from build123d import *

# Parameters (mm, degrees)
SKETCH1_R           = 12.7
BOSS_EXTRUDE1_DEPTH = 12.7
SKETCH1_3_R         = 3.175
BOSS_EXTRUDE2_DEPTH = 6.35
SKETCH1_4_R         = 3.175
BOSS_EXTRUDE3_DEPTH = 99.06


with BuildPart() as part:
    # Sketch1 → Boss-Extrude1 (new body)
    with BuildSketch(Plane.XY):
        Circle(SKETCH1_R)
    extrude(amount=-BOSS_EXTRUDE1_DEPTH)

    # Sketch1<3> → Boss-Extrude2 (add)
    with BuildSketch(Plane.XY):
        with BuildLine():
            Line((9.391776656, -58.7375), (18.783553311, -3.175))
            ThreePointArc((18.783553311, -3.175), (0, 19.05), (-18.783553311, -3.175))
            Line((-18.783553311, -3.175), (-9.391776656, -58.7375))
            ThreePointArc((-9.391776656, -58.7375), (0, -66.675), (9.391776656, -58.7375))
        make_face()
        with Locations((0, -57.15)):
            Circle(SKETCH1_3_R, mode=Mode.SUBTRACT)
    extrude(amount=BOSS_EXTRUDE2_DEPTH)

    # Sketch1<4> → Boss-Extrude3 (add)
    with BuildSketch(Plane.XY):
        with Locations((0, -57.15)):
            Circle(SKETCH1_4_R)
    extrude(amount=BOSS_EXTRUDE3_DEPTH)


solid = part.part
Design review of the part built by this model. Coordinates are the model's own, in mm. A direction names the side the tool comes from. Give positions to 0.01 mm unless a question says otherwise; leave off trailing zeros. Order: outer loops, then holes, each group sorted by start corner. A loop starts at its lowest first (then second) coordinate and runs counter-clockwise, first axis right, second up.
1. Add section A-A, the plane x = 0. State the section outline as (y, z) points (3 decimals), then the cut area to 3 significant figures.
Solution:
outline: (-66.675, 0) - (-12.7, 0) - (-12.7, -12.7) - (12.7, -12.7) - (12.7, 0) - (19.05, 0) - (19.05, 6.35) - (-53.975, 6.35) - (-53.975, 99.06) - (-60.325, 99.06) - (-60.325, 6.35) - (-66.675, 6.35) - close
area: 1,460 mm2
2. Add section B-B, the plane y = 0. State the section outline as (x, z) points, then the cut area to 3 significant figures.
Solution:
outline: (-19.05, 0) - (-12.7, 0) - (-12.7, -12.7) - (12.7, -12.7) - (12.7, 0) - (19.05, 0) - (19.05, 6.35) - (-19.05, 6.35) - close
area: 565 mm2
3. Add section C-C, the plane z = 77. State the section outline as (x, y) points (3 decimals), then the cut area to 3 significant figures.
Solution:
outline: circle Ø6.35 at (0, -57.15)
area: 31.7 mm2
4. To check wall thickness, follow L1, parallel to Z at x = 6.5, y = -62.5; L2, parallel to X at y = 1, z = 4; L3, parallel to Y at x = 4.5, z = 2. State the ranges of each line that lie inside material, in increasing order.
Solution:
L1: z = 0 to 6.35
L2: x = -19.02 to 19.02
L3: y = -65.54 to 18.51
5. Tool access review of faces 1 (the flat face through (-14.153, -30.567, 3.131)), 2 (the cylindrical face through (1.707, -54.473, 52.056)), 3 (the cylindrical face through (-2.75, -12.4, -6.26)): name each direction out of +Z, -Z, +X, -X, +Y, -Y from which nothing blocks a thin tool from reaching the whole face with its end or side.
Solution:
face 1: +Z, -Z, -X, -Y
face 2: +Z
face 3: -Z
6. Add section D-D, the plane x = 11.5. State the section outline as (y, z) points, then the cut area to 3 significant figures.
Solution:
outline: (-46.27, 0) - (-5.39, 0) - (-5.39, -12.7) - (5.39, -12.7) - (5.39, 0) - (15.19, 0) - (15.19, 6.35) - (-46.27, 6.35) - close
area: 527 mm2
7. For pin 1 Ø19 at (x, y) = (8.5, -18.5) entering from +Z, flat-tipped, find the tip position at first contact; note if it passes through.
Solution:
pin 1: stops at z = 6.35
